```python
from build123d import *

# Parameters (mm, degrees)
EXTRUDE_1_DEPTH        = 11
SKETCH_6_R             = 5
CUT_EXTRUDE_2_DEPTH    = 15
SKETCH_7_R             = 2.75
CUT_EXTRUDE_3_DEPTH    = 6
EXTRUDE_START          = 10
SKETCH_18_R            = 14
SKETCH_18_R_2          = 7
EXTRUDE_2_DEPTH        = 10
HOLE_WIZARD_M5_2_D     = 4.2
HOLE_WIZARD_M5_2_DEPTH = 19
HOLE_WIZARD_M5_2_TIP   = 1.2618073


with BuildPart() as part:
    # 草图1 → 凸台-拉伸1 (new body)
    with BuildSketch(Plane.XY):
        with BuildLine():
            Line((-13.964240044, 1), (-6.92820323, 1))
            ThreePointArc((-6.92820323, 1), (6.998743905, -0.13260372), (-6.96111081, -0.736842105))
            Line((-6.96111081, -0.736842105), (-13.982489049, -0.7))
            ThreePointArc((-13.982489049, -0.7), (13.999193432, -0.150277266), (-13.964240044, 1))
        make_face()
    extrude(amount=EXTRUDE_1_DEPTH)

    # 切除-扫描1: sweep along a path in 草图3
    with BuildLine(Plane(origin=(0, 0, 0), x_dir=(1, 0, 0), z_dir=(0, 1, 0))) as sweep_1_path:
        Line((11.898777818, -11), (9.4677896, -8.569011782))
    # 草图2 → 切除-扫描1 (sweep, cut)
    with BuildSketch(Plane.XY.offset(11)):
        with BuildLine():
            Line((6.981701169, 0.505814966), (11.898777818, 0.505814966))
            Line((11.898777818, 0.505814966), (11.898777818, -0.505814966))
            Line((11.898777818, -0.505814966), (6.981701169, -0.505814966))
            ThreePointArc((6.981701169, -0.505814966), (7, 0), (6.981701169, 0.505814966))
        make_face()
    sweep(path=sweep_1_path.line, mode=Mode.SUBTRACT)

    # 草图6 → 切除-拉伸2 (cut)
    with BuildSketch(Plane(origin=(0, 6, 0), x_dir=(1, 0, 0), z_dir=(0, 1, 0))):
        with Locations((-9.464240044, -5.5)):
            Circle(SKETCH_6_R)
    extrude(amount=CUT_EXTRUDE_2_DEPTH, mode=Mode.SUBTRACT)

    # 草图7 → 切除-拉伸3 (cut)
    with BuildSketch(Plane(origin=(0, 6, 0), x_dir=(1, 0, 0), z_dir=(0, 1, 0))):
        with Locations(Location((-9.464240044, -5.5, 0), (0, 0, 270))):
            Circle(SKETCH_7_R)
    extrude(amount=-CUT_EXTRUDE_3_DEPTH, mode=Mode.SUBTRACT)

    # 草图18 → 凸台-拉伸2 (add)
    with BuildSketch(Plane(origin=(0, 0, 0), x_dir=(-1, 0, 0), z_dir=(0, 0, -1)).offset(EXTRUDE_START)):
        Circle(SKETCH_18_R)
        Circle(SKETCH_18_R_2, mode=Mode.SUBTRACT)
    extrude(amount=-EXTRUDE_2_DEPTH)

    # M5 螺纹孔2
    with Locations(Plane(origin=(-0.004057853, -0.773346687, 0), x_dir=(0.9999862340820442, -0.005247060740183186, 0), z_dir=(0.005247060740183185, 0.9999862340820441, 0))):
        with Locations((-9.411026536, -5.540271142)):
            Hole(HOLE_WIZARD_M5_2_D / 2, depth=HOLE_WIZARD_M5_2_DEPTH)
            with Locations((0, 0, -(HOLE_WIZARD_M5_2_DEPTH + HOLE_WIZARD_M5_2_TIP / 2))):  # 118° drill point
                Cone(0, HOLE_WIZARD_M5_2_D / 2, HOLE_WIZARD_M5_2_TIP, mode=Mode.SUBTRACT)


solid = part.part
```
The listing builds one solid part. Answer for the finished solid, in the listing's coordinates (mm). A direction names the side the tool comes from. Round coordinates to 2 decimals unless told otherwise and drop trailing zeros. Order: outer loops, then holes, each group sorted by start corner. A loop starts at its lowest first (then second) coordinate and runs counter-clockwise, first axis right, second up. Notation, with made-up numbers: (82.25, 89) -> (98.25, 89) arc R21 cw to (98.25, 107) -> close; hole circle Ø6 at (8, 16). An arc over 180 degrees is marked (long way). Answer as CSV lines item,"result". Start each with the question number.
(1) The part is cut by section D-D (y = 11.25). Determine the outline of the cut face in (x, z), then the cut area to 3 significant figures.
(2) A tool of negligible diameter and unlimited length cuts with its end or side. For faces 1 (the face through (6.4, 3.3, -10)), 2 (the face through (-7.34, -5.16, 5.45)), 3 (the face through (10.7, 0, 9.8)), 4 (the face through (-11.904, 3.535, 6.769)), from which of +Z, -Z, +X, -X, +Y, -Y can it reach the whole face along a straight path? Write none if from no direction.
(3) Find the intervals of material crossed by probe 1 along Y at (x, z) = (0, 3.5); probe 2 along X at (y, z) = (0, 6.25); probe 3 along X at (y, z) = (4.75, 8.5), in increasing order. Write a range as from..to.
(4) The part is cut by section A-A (x = 0). Determine the outline of the cut face in (y, z), then the cut area to 3 significant figures.
(5) The part is cut by section B-B (y = 0). Determine the outline of the cut face in (x, z), then the cut area to 3 significant figures.
(6) For a pull along Y with two mould halves and no side action, classify faces 5 (the face through (-6.4, 3.3, 11)), 6 (the face through (-6.8, 6, 4.3)), 7 (the face through (9, 0.506, 10)) as +Y half, -Y half, draft (parallel to the pull), parting line (faces both ways), or undercut.
(7) Flat-ended cylindrical pins translate along their axes: pin 1 Ø8 at (y, z) = (4.5, 9) entering from +X; pin 2 Ø11.5 at (x, z) = (-9.46, 5.5) entering from -Y; pin 3 Ø1.2 at (x, z) = (9.5, 9.5) entering from +Y; pin 4 Ø11 at (x, y) = (0, 0) entering from -Z. Find the tip coordinate at first contact, or state that the pin passes through.
(8) The part is cut by section C-C (z = -0.5). Determine the outline of the cut face in (x, y).
Evaluation:
1,outline,"(-8.33, -10) -> (8.33, -10) -> (8.33, 11) -> (-8.33, 11) -> (-8.33, 10.37) arc R5 cw to (-8.33, 0.63) -> close"
1,area,"322 mm²"
2,face 1,"-Z, +X, -X, +Y, -Y"
2,face 2,"none"
2,face 3,"+Z, -X"
2,face 4,"+Y"
3,probe 1,"-14..-7, 7..14"
3,probe 2,"7..14"
3,probe 3,"-13.17..-5.14, 5.14..13.17"
4,outline,"(-14, -10) -> (-7, -10) -> (-7, 11) -> (-14, 11) -> close; (7, -10) -> (14, -10) -> (14, 11) -> (7, 11) -> close"
4,area,"294 mm²"
5,outline,"(-14, -10) -> (-7, -10) -> (-7, 0) -> (-14, 0) -> close; (7, -10) -> (14, -10) -> (14, 11) -> (11.9, 11) -> (9.47, 8.57) -> (7, 8.57) -> close"
5,area,"208 mm²"
6,face 5,"draft"
6,face 6,"+Y half"
6,face 7,"undercut"
7,pin 1,"x = 13.99"
7,pin 2,"y = -13.5"
7,pin 3,"y = 10.81"
7,pin 4,"through"
8,outline,"circle Ø28 at (0, 0); hole circle Ø14 at (0, 0)"
